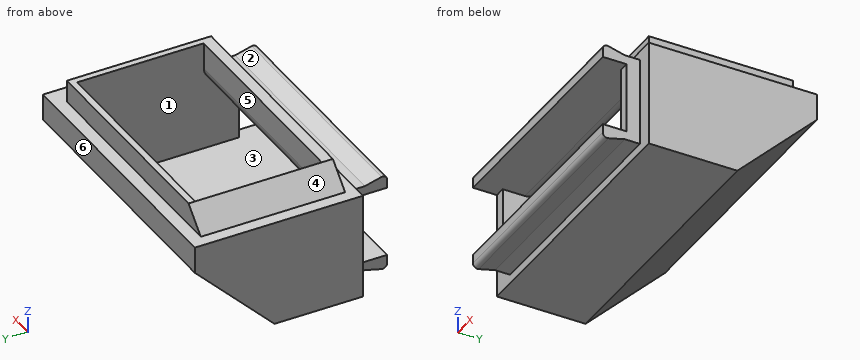
from build123d import *

# Parameters (mm, degrees)
SKETCH1_W           = 31
SKETCH1_H           = 12
BOSS_EXTRUDE1_DEPTH = 19
SKETCH2_W           = 24.1
SKETCH2_H           = 8
CUT_EXTRUDE1_DEPTH  = 16.8
SKETCH3_W           = 24.1
SKETCH3_H           = 14.3
CUT_EXTRUDE2_DEPTH  = 2
FILLET1_SIZE        = 8
FILLET2_SIZE        = 9
SKETCH6_W           = 26.5
SKETCH6_H           = 1
BOSS_EXTRUDE3_DEPTH = 4.2
BOSS_EXTRUDE6_DEPTH = 26.5
SKETCH15_W          = 1.2
SKETCH15_H          = 8
BOSS_EXTRUDE7_DEPTH = 1.5
SKETCH4_W           = 27.35
SKETCH4_H           = 16.3
SKETCH4_W_2         = 24.1
SKETCH4_H_2         = 14.3
BOSS_EXTRUDE2_DEPTH = 2.5
CHAMFER1_SIZE       = 2.5
FILLET3_R           = 1.5


with BuildPart() as part:
    # Sketch1 → Boss-Extrude1 (new body)
    with BuildSketch(Plane(origin=(0, 0, 0), x_dir=(1, 0, 0), z_dir=(0, 1, 0))):
        Rectangle(SKETCH1_W, SKETCH1_H)
    extrude(amount=BOSS_EXTRUDE1_DEPTH)

    # Sketch2 → Cut-Extrude1 (cut)
    with BuildSketch(Plane.XZ):
        with Locations((0.45, 0)):
            Rectangle(SKETCH2_W, SKETCH2_H)
    extrude(amount=-CUT_EXTRUDE1_DEPTH, mode=Mode.SUBTRACT)

    # Sketch3 → Cut-Extrude2 (cut)
    with BuildSketch(Plane.XY.offset(6)):
        with Locations((0.45, 9.65)):
            Rectangle(SKETCH3_W, SKETCH3_H)
    extrude(amount=-CUT_EXTRUDE2_DEPTH, mode=Mode.SUBTRACT)

    # Fillet1
    fillet1_edges = [part.edges().sort_by_distance(p)[0] for p in [
        (0.45, 16.8, -4),
    ]]
    chamfer(fillet1_edges, length=FILLET1_SIZE)

    # Fillet2
    fillet2_edges = [part.edges().sort_by_distance(p)[0] for p in [
        (0, 19, -6),
    ]]
    chamfer(fillet2_edges, length=FILLET2_SIZE)

    # Sketch6 → Boss-Extrude3 (add)
    with BuildSketch(Plane.XZ):
        with Locations((0.45, 4.5)):
            Rectangle(SKETCH6_W, SKETCH6_H)
        with Locations((0.45, -4.5)):
            Rectangle(SKETCH6_W, SKETCH6_H)
    extrude(amount=BOSS_EXTRUDE3_DEPTH)

    # Sketch14 → Boss-Extrude6 (add)
    with BuildSketch(Plane(origin=(13.7, 0, 0), x_dir=(0, 0, -1), z_dir=(1, 0, 0))):
        with BuildLine():
            Line((5.484122918, -3.575), (5, -1.7))
            Line((5, -1.7), (5, -4.2))
            ThreePointArc((5, -4.2), (5.395284708, -4.006186218), (5.484122918, -3.575))
        make_face()
        with BuildLine():
            Line((-5, -4.2), (-5, -1.7))
            Line((-5, -1.7), (-5.484122918, -3.575))
            ThreePointArc((-5.484122918, -3.575), (-5.395284708, -4.006186218), (-5, -4.2))
        make_face()
    extrude(amount=-BOSS_EXTRUDE6_DEPTH)

    # Sketch15 → Boss-Extrude7 (add)
    with BuildSketch(Plane.XZ):
        with Locations((-12.2, 0)):
            Rectangle(SKETCH15_W, SKETCH15_H)
        with Locations((13.1, 0)):
            Rectangle(SKETCH15_W, SKETCH15_H)
    extrude(amount=BOSS_EXTRUDE7_DEPTH)

    # Sketch4 → Boss-Extrude2 (add)
    with BuildSketch(Plane.XY.offset(6)):
        with Locations((-0.425, 9.4)):
            Rectangle(SKETCH4_W, SKETCH4_H)
        with Locations((0.45, 9.65)):
            Rectangle(SKETCH4_W_2, SKETCH4_H_2, mode=Mode.SUBTRACT)
    extrude(amount=BOSS_EXTRUDE2_DEPTH)

    # Chamfer1
    chamfer1_edges = [part.edges().sort_by_distance(p)[0] for p in [
        (-14.1, 9.4, 8.5),
    ]]
    chamfer(chamfer1_edges, length=CHAMFER1_SIZE - 0.0001)  # a hair under: the kernel refuses the full size

    # Fillet3
    fillet3_edges = [part.edges().sort_by_distance(p)[0] for p in [
        (0.45, 2.5, 4),
    ]]
    fillet(fillet3_edges, radius=FILLET3_R)


solid = part.part
Verification items for the finished model (mm, model axes). Face numbers are marked on the shaded views. A direction names the side the tool comes from. Give positions to 0.01 mm unless a question says otherwise; leave off trailing zeros. Order: outer loops, then holes, each group sorted by start corner. A loop starts at its lowest first (then second) coordinate and runs counter-clockwise, first axis right, second up. Notation, with made-up numbers: M 12,6 L 52,6 A33 cw 52,42 Z; hole C -32.75,-8 d2. An arc over 180 degrees is marked long. Answer as a JSON object with one key per item and string values. Group by question number.
1) Depth check by flat-ended pin: pin 1 Ø1.5 at (x, z) = (5, -2) entering from +Y; pin 2 Ø0.8 at (y, z) = (10.5, 7.5) entering from +X; pin 3 Ø1.5 at (x, z) = (3, 7) entering from +Y. Enter the tip coordinate at first touch or a pass-through.
2) Scan lines: line 1 along Z through (x, y) = (0, -1.5); line 2 along Y through (x, z) = (0.5, 7.75); line 3 along X through (y, z) = (7.5, 1.25). Record each from-to range of solid material in increasing order. Write a range as [from, to].
3) Cross-section at C-C (z = -2.25). Enter the section's corners in (x, y), then the cut area to 3 significant figures.
4) Mould release check, pull along X, two halves, no side actions. Record for the marked faces 4, 5 and 6: released by +X, released by -X, zero draft, split by the parting line, or undercut.
5) Cross-section at B-B (y = -0.5). Enter the section's corners in (x, z), then the cut area to 3 significant figures.
6) Access from +Z, -Z, +X, -X, +Y, -Y to the whole of each face (thin tool, end or side, straight path). Record for the marked faces 1, 2 and 3.
7) Cross-section at A-A (x = 11.5). Enter the section's corners in (y, z) (3 decimals), then the cut area to 3 significant figures.
Result sheet:
{
 "1": {"pin 1": "stops at y = 14.75", "pin 2": "stops at x = 13.25", "pin 3": "stops at y = 17.55"},
 "2": {"line 1": "z = [-5, -4], [4, 5]", "line 2": "y = [1.25, 2.5], [16.8, 17.55]", "line 3": "x = [-15.5, -11.6], [12.5, 15.5]"},
 "3": {"outline": "M -15.5,0 L -12.8,0 L -12.8,-1.5 L -11.6,-1.5 L -11.6,10.55 L 12.5,10.55 L 12.5,-1.5 L 13.7,-1.5 L 13.7,0 L 15.5,0 L 15.5,13.75 L -15.5,13.75 Z", "area": "176 mm2"},
 "4": {"face 4": "released by -X", "face 5": "undercut", "face 6": "zero draft"},
 "5": {"outline": "M -12.8,-5 L 13.7,-5 L 13.7,5 L -12.8,5 Z; hole M -11.6,-4 L 12.5,-4 L 12.5,4 L -11.6,4 Z", "area": "72.2 mm2"},
 "6": {"face 1": "none", "face 2": "+Z, +X, -X", "face 3": "-Y"},
 "7": {"outline": "M -4.2,-5 A0.5 ccw -3.575,-5.484 L -1.7,-5 L 0,-5 L 0,-6 L 10,-6 L 19,3 L 19,6 L 17.55,6 L 17.55,8.5 L 16.8,8.5 L 16.8,4 L 8.8,-4 L -4.2,-4 Z; M -4.2,4 L 1,4 A1.5 ccw 2.5,5.5 L 2.5,8.5 L 1.25,8.5 L 1.25,6 L 0,6 L 0,5 L -1.7,5 L -3.575,5.484 A0.5 ccw -4.2,5 Z", "area": "70.8 mm2"}
}
